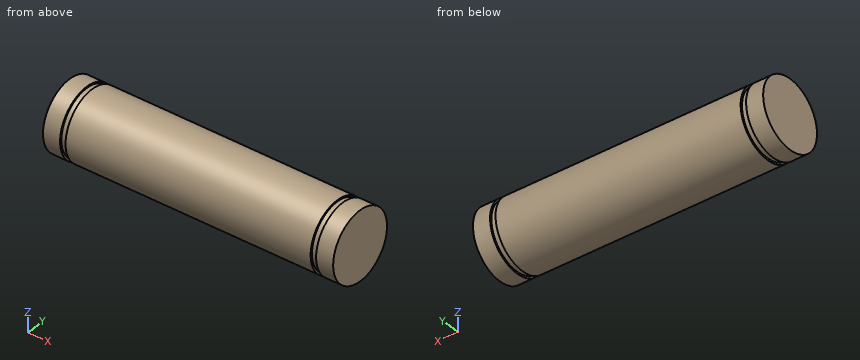
from build123d import *

# Parameters (mm, degrees)
SKETCH1_R           = 2
BOSS_EXTRUDE1_DEPTH = 17
SKETCH3_W           = 0.483504557
SKETCH3_H           = 0.32
SKETCH3_W_2         = 1.446691601


with BuildPart() as part:
    # Sketch1 → Boss-Extrude1 (new body)
    with BuildSketch(Plane(origin=(0, 0, 0), x_dir=(0, 0, -1), z_dir=(1, 0, 0))):
        Circle(SKETCH1_R)
    extrude(amount=BOSS_EXTRUDE1_DEPTH)

    # Sketch3 → Groove for ANSI B27.7 - 3AM1-4, Basic External Retaining Ring1 (revolve, cut)
    with BuildSketch(Plane(origin=(15, 0, 0), x_dir=(0, 0, 1), z_dir=(0, -1, 0))):
        with Locations((2.158247722, -0.84)):
            Rectangle(SKETCH3_W, SKETCH3_H)
        with Locations((2.639841244, 13.84)):
            Rectangle(SKETCH3_W_2, SKETCH3_H)
    revolve(axis=Axis((67.749749937, 0, 0.016495443), (-1, 0, 0)), mode=Mode.SUBTRACT)


solid = part.part
Design review of the part built by this model. Coordinates are the model's own, in mm. Give positions to 0.01 mm unless a question says otherwise; leave off trailing zeros. Write each loop counter-clockwise with the first axis right and the second up, starting at its lowest first coordinate (ties: lowest second). Pieces come first, ordered by that corner, then holes. Notation, with made-up numbers: M 76,-11.5 L 82,-11.5 A18 cw 82,14.5 Z; hole C 43.25,3 d3. An arc over 180 degrees is marked long. Answer as a JSON object with one key per item and string values. Group by question number.
1) For line 1 along Z through (x, y) = (13.25, -0.1); line 2 along Y through (x, z) = (14, 0.35); line 3 along Z through (x, y) = (10.5, 1.1), list the stretches that pass through material, from the lowest coordinate up.
2) We need section B-B (y = -0.8). Give the boundary of the cut face in (x, z).
3) We need section C-C (x = 9.25). Give the boundary of the cut face in (y, z), and give its area (3 significant figures).
4) Clearance check with a flat-ended pin moving along its axis: pin 1 Ø1 at (x, y) = (10, -0.5) entering from +Z. State where the tip first meets the part, or that it passes through.
5) We need section A-A (z = 1.6). Give the boundary of the cut face in (x, y), and give its area (3 significant figures).
Answer key:
{
 "1": {"line 1": "z = -2 to 2", "line 2": "y = -1.97 to 1.97", "line 3": "z = -1.67 to 1.67"},
 "2": {"outline": "M 0,-1.83 L 1,-1.83 L 1,-1.71 L 1.32,-1.71 L 1.32,-1.83 L 15.68,-1.83 L 15.68,-1.71 L 16,-1.71 L 16,-1.83 L 17,-1.83 L 17,1.83 L 16,1.83 L 16,1.74 L 15.68,1.74 L 15.68,1.83 L 1.32,1.83 L 1.32,1.74 L 1,1.74 L 1,1.83 L 0,1.83 Z"},
 "3": {"outline": "C 0,0 d4", "area": "12.6 mm²"},
 "4": {"pin 1": "stops at z = 2"},
 "5": {"outline": "M 0,-1.2 L 1,-1.2 L 1,-1.05 L 1.32,-1.05 L 1.32,-1.2 L 15.68,-1.2 L 15.68,-1.05 L 16,-1.05 L 16,-1.2 L 17,-1.2 L 17,1.2 L 16,1.2 L 16,1.05 L 15.68,1.05 L 15.68,1.2 L 1.32,1.2 L 1.32,1.05 L 1,1.05 L 1,1.2 L 0,1.2 Z", "area": "40.6 mm²"}
}
